Design review of the part shown in the three views and the two pictorial views. Dimensions are in mm from the part's minimum x, y and z. A direction names the side the tool comes from. Round coordinates to 2 decimals unless told otherwise and drop trailing zeros. Loops run counter-clockwise (first coordinate to the right, second up) from the corner with the lowest first, then second, coordinate; pieces in that order, holes last.
1) Take a section at B-B (x = 3.5). State the section outline as (y, z) points.
2) Take a section at A-A (y = 8.75). State the section outline as (x, z) points.
3) Tool access review of the marked faces 1 and 2: name each direction out of +Z, -Z, +X, -X, +Y, -Y from which nothing blocks a thin tool from reaching the whole face with its end or side.
4) Take a section at C-C (z = 0.75). State the section outline as (x, y) points.
5) Wall thickness on L1, parallel to Z at x = 1.25, y = 8; L2, parallel to X at y = 5.5, z = 8: over which ranges is each line inside the solid? List them lowest first.
6) Insertion check: pin 1 (4 mm diameter, centred on x = 4, y = 5, fed in from -Z); pin 2 (4 mm diameter, centred on y = 4.5, z = 5.5, fed in from -X). Each pin has a flat end and moves straight along its axis. Give the tip position at first contact, or say it passes through.
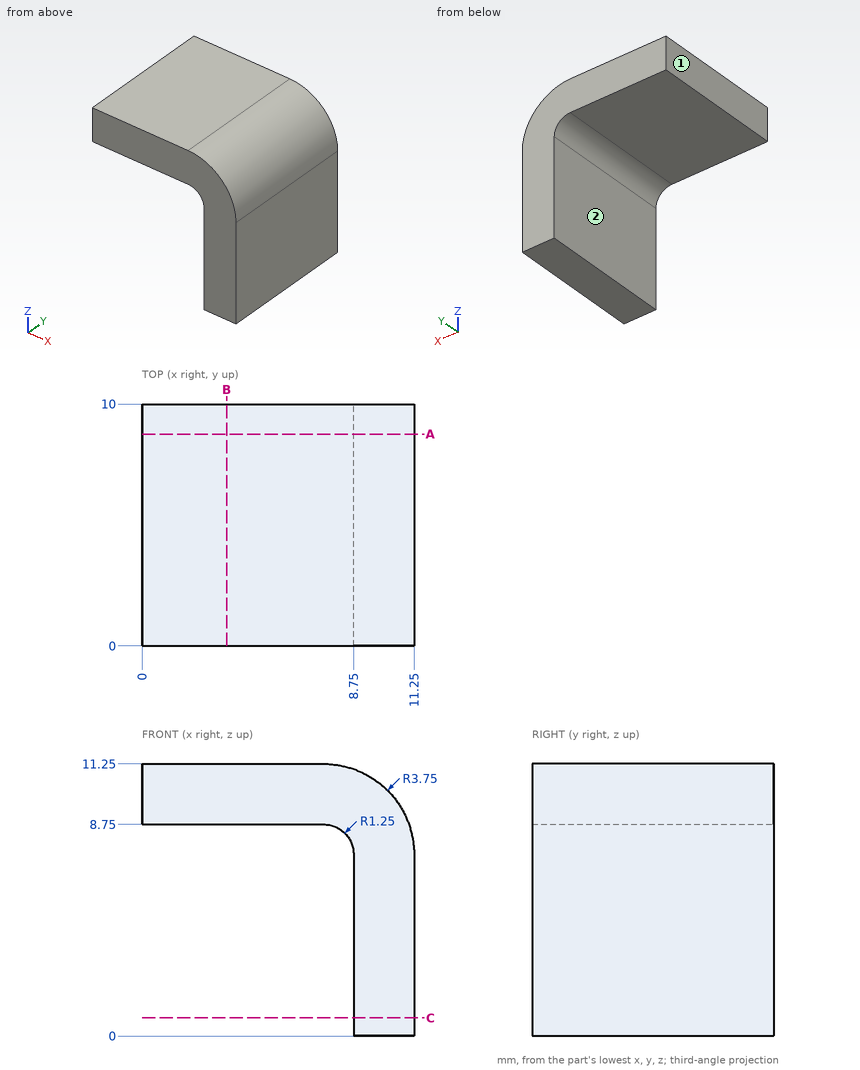
Response:
1. outline: (0, 8.75) - (10, 8.75) - (10, 11.25) - (0, 11.25) - close
2. outline: (0, 8.75) - (7.5, 8.75) arc R1.25 cw to (8.75, 7.5) - (8.75, 0) - (11.25, 0) - (11.25, 7.5) arc R3.75 ccw to (7.5, 11.25) - (0, 11.25) - close
3. face 1: +Z, -Z, -X, +Y, -Y
3. face 2: -Z, -X, +Y, -Y
4. outline: (8.75, 0) - (11.25, 0) - (11.25, 10) - (8.75, 10) - close
5. L1: z = 8.75 to 11.25
5. L2: x = 8.65 to 11.22
6. pin 1: stops at z = 8.75
6. pin 2: stops at x = 8.75
